Work out the finished part from the listing and answer in its coordinate system (mm). A direction names the side the tool comes from. Coordinates: 2 decimals unless noted, no trailing zeros. Order: outer loops, then holes, each group sorted by start corner. A loop starts at its lowest first (then second) coordinate and runs counter-clockwise, first axis right, second up. Notation, with made-up numbers: M 75.25,77.5 L 129.25,77.5 A18 cw 129.25,107.5 Z; hole C -15.75,71 d11. An arc over 180 degrees is marked long. Write item = value, one per line. Start each with the question number.
Q1. A tool of negligible diameter and unlimited length cuts with its end or side. For faces 1 (the cylindrical face through (25.2, 5.05, 1.36)), 2 (the flat face through (14, 11, 0)), 3 (the flat face through (14, 0, 2)), from which of +Z, -Z, +X, -X, +Y, -Y can it reach the whole face along a straight path? Write none if from no direction.
Q2. Straight lines are drawn through the part: line 1 along Y through (x, z) = (24, 2.05); line 2 along X through (y, z) = (4.5, 3.15); line 3 along X through (y, z) = (6, 0.6). For each, find the intervals that lie inside material, in ascending order.
Q3. Find section C-C on z = 1.5. Give the vertices of the cut face in (x, y).
Q4. Determine the mould class of faces 4 (the flat face through (14, 10, 2)), 5 (the flat face through (0, 5, 1)), 6 (the cylindrical face through (5.2, 5.05, 1.36)) for opening direction X: released by +X, released by -X, zero draft, split by the parting line, or undercut.
Q5. Each of these flat-tipped pins is pushed along its axis until it touches: P1, Ø1.2, axis at x = 14, z = 1.5, coming from the +Y side; P2, Ø1.4, axis at x = 24, y = 5, coming from the +Z side; P3, Ø2, axis at x = 18.5, z = 1.5, coming from the -Y side. Where does it stop, or does it pass through?
Q6. Find section D-D on x = 9.75. Give the vertices of the cut face in (y, z).
Q7. Find section B-B on y = 5. Give the vertices of the cut face in (x, z).
Q8. Find section A-A on x = 24. Give the vertices of the cut face in (y, z), and give its area (3 significant figures).
```python
from build123d import *

# Parameters (mm, degrees)
F0_W          = 28
F0_H          = 4
F1_DEPTH      = 10
F2_W          = 28
F2_H          = 1.2
F3_DEPTH      = 1.2
F3_DEPTH_BACK = 11.2
F5_D          = 2.4
F5_DEPTH      = 15


with BuildPart() as f1:
    # F0 (on Front) → F1 (new body)
    with BuildSketch(Plane.XZ):
        with Locations((14, 2)):
            Rectangle(F0_W, F0_H)
    extrude(amount=-F1_DEPTH)

    # F2 (on Front) → F3 (join, two sides)
    with BuildSketch(Plane.XZ) as f3_sk:
        with Locations((14, -0.6)):
            Rectangle(F2_W, F2_H)
    extrude(amount=F3_DEPTH)
    extrude(f3_sk.sketch, amount=-F3_DEPTH_BACK)

    # F5
    with Locations(Plane.XY.offset(4)):
        with Locations((4, 5), (24, 5)):
            Hole(F5_D / 2, depth=F5_DEPTH)


solid = f1.part
```
Findings below:
q1.face_1 = +Z, -Z
q1.face_2 = +Z, +X, -X, +Y
q1.face_3 = +Z, +X, -X, -Y
q2.line_1 = 0 to 3.8, 6.2 to 10
q2.line_2 = 0 to 2.91, 5.09 to 22.91, 25.09 to 28
q2.line_3 = 0 to 3.34, 4.66 to 23.34, 24.66 to 28
q3.outline = M 0,0 L 28,0 L 28,10 L 0,10 Z; hole C 4,5 d2.4; hole C 24,5 d2.4
q4.face_4 = zero draft
q4.face_5 = released by -X
q4.face_6 = undercut
q5.P1 = 10
q5.P2 = through
q5.P3 = 0
q6.outline = M -1.2,-1.2 L 11.2,-1.2 L 11.2,0 L 10,0 L 10,4 L 0,4 L 0,0 L -1.2,0 Z
q7.outline = M 0,-1.2 L 2.8,-1.2 L 2.8,4 L 0,4 Z; M 5.2,-1.2 L 22.8,-1.2 L 22.8,4 L 5.2,4 Z; M 25.2,-1.2 L 28,-1.2 L 28,4 L 25.2,4 Z
q8.outline = M -1.2,-1.2 L 3.8,-1.2 L 3.8,4 L 0,4 L 0,0 L -1.2,0 Z; M 6.2,-1.2 L 11.2,-1.2 L 11.2,0 L 10,0 L 10,4 L 6.2,4 Z
q8.area = 42.4 mm^2
